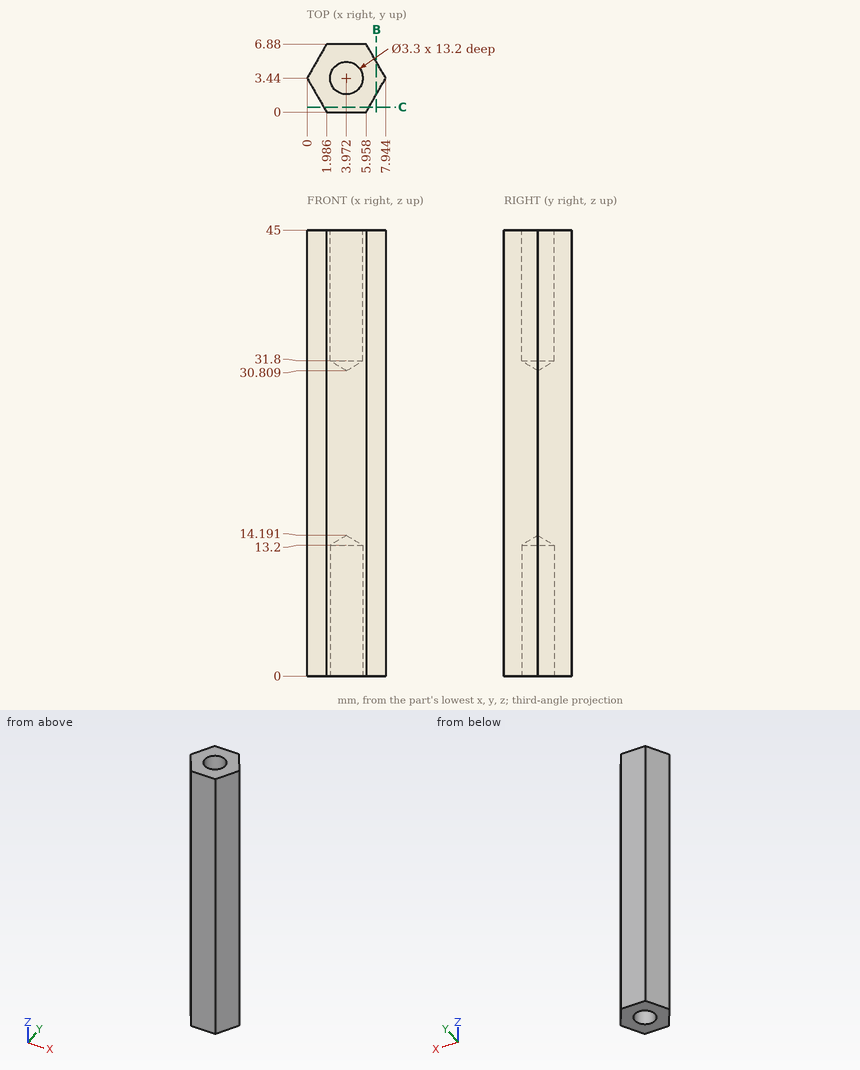
Geometry: see drawing. Coordinates: mm, zero at the bounding-box minimum. Coordinates: 2 decimals unless noted, no trailing zeros. Write each loop counter-clockwise with the first axis right and the second up, starting at its lowest first coordinate (ties: lowest second). Pieces come first, ordered by that corner, then holes.
1) Material intervals for line 1 along X through (y, z) = (3.44, 36.25) (1 decimal); line 2 along X through (y, z) = (4.25, 2) (1 decimal); line 3 along Y through (x, z) = (2.75, 10), sorted ascending.
2) Section C-C on y = 0.5. Output: boundary loops of the cut face in (x, z), and give its area (3 significant figures).
3) Section B-B on x = 7. Output: boundary loops of the cut face in (y, z) (1 decimal), and give its area (3 significant figures).
4) Pin query (flat end, axial travel): pin 1 Ø2.5 at (x, y) = (3.97, 3.44) entering from +Z; pin 2 Ø3 at (y, z) = (3.5, 21) entering from +X; pin 3 Ø2 at (y, z) = (6, 5.5) entering from -X. Return the tip coordinate at first contact, or that it passes through.
Check result:
1. line 1: x = 0 to 2.3, 5.6 to 7.9
1. line 2: x = 0.5 to 2.5, 5.4 to 7.5
1. line 3: y = 0 to 2.33, 4.55 to 6.88
2. outline: (1.7, 0) - (6.25, 0) - (6.25, 45) - (1.7, 45) - close
2. area: 205 mm2
3. outline: (1.8, 0) - (5.1, 0) - (5.1, 45) - (1.8, 45) - close
3. area: 147 mm2
4. pin 1: stops at z = 31.56
4. pin 2: stops at x = 7.94
4. pin 3: stops at x = 0.9
